For this review, take the finished solid that the model builds, in its own axes (mm). Face numbers are marked on the shaded views. Give positions to 0.01 mm unless a question says otherwise; leave off trailing zeros. Order: outer loops, then holes, each group sorted by start corner. A loop starts at its lowest first (then second) coordinate and runs counter-clockwise, first axis right, second up. Notation, with made-up numbers: (79.5, 35.25) - (126.5, 35.25) arc R30 ccw to (126.5, 66.25) - close; hole circle Ø5 at (-5, -29.75). An arc over 180 degrees is marked (long way). Put each result on its own line as item: value. Start each with the question number.
```python
from build123d import *

# Parameters (mm, degrees)
SKETCH1_R           = 12.35
BOSS_EXTRUDE1_DEPTH = 25
CIRPATTERN1_COUNT   = 4
SKETCH7_W           = 3.7
SKETCH7_H           = 1.9


with BuildPart() as part:
    # Sketch1 → Boss-Extrude1 (new body)
    with BuildSketch(Plane.XY):
        Circle(SKETCH1_R)
    extrude(amount=BOSS_EXTRUDE1_DEPTH)

    # Sketch2 → M4x0.7 Tapped Hole1 (revolve, cut)
    with BuildSketch(Plane(origin=(-0.784484958, 12.325059162, 10), x_dir=(-0.9979804989599389, -0.06352104923308127, 0), z_dir=(0, 0, 1))):
        Polygon((0, 0), (0, 9.991420021), (1.65, 9), (1.65, 0.85), (2.5, 0), align=None)
    m4x0_7_tapped_hole1 = revolve(axis=Axis((-1.187843621, 18.662235331, 10), (0.06352104923308129, -0.9979804989599389, 0)), mode=Mode.SUBTRACT)

    # CirPattern1: M4x0.7 Tapped Hole1 ×4 about axis
    cirpattern1_axis = Axis((0, 0, 25), (0, 0, -1))
    for i in range(1, CIRPATTERN1_COUNT):
        add(m4x0_7_tapped_hole1.rotate(cirpattern1_axis, i * 360 / CIRPATTERN1_COUNT), mode=Mode.SUBTRACT)

    # Sketch7 → Cut-Revolve1 (revolve, cut)
    with BuildSketch(Plane(origin=(0, 0, 0), x_dir=(0, 0, -1), z_dir=(1, 0, 0)), mode=Mode.PRIVATE) as cut_revolve1_sk:
        with Locations((-16.85, 11.4)):
            Rectangle(SKETCH7_W, SKETCH7_H)
    revolve(cut_revolve1_sk.sketch.rotate(Axis((0, 0, 25), (0, 0, -1)), 90), axis=Axis((0, 0, 25), (0, 0, -1)), mode=Mode.SUBTRACT)


solid = part.part
```
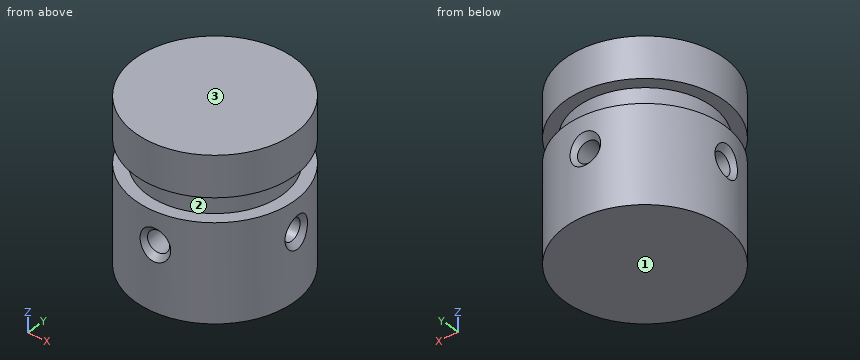
1. The part is to be moulded in two halves that separate along Z. For the marked faces 1, 2 and 3, say which applies: released by +Z, released by -Z, zero draft, split by the parting line, or undercut.
2. Clearance check with flat-ended pins moving along their axes: pin 1 (1.5 mm diameter, centred on x = -6.5, z = 7.5, fed in from -Y); pin 2 (1 mm diameter, centred on x = -9, z = 9.5, fed in from -Y); pin 3 (6 mm diameter, centred on x = 5.5, z = 17, fed in from +Y). State where each tip first meets the part, or that it passes through.
3. Wall thickness on line 1 (Z direction, x = 11, y = -5); line 2 (Z direction, x = -11, y = -0.5); line 3 (Z direction, x = 1, y = -4): over which ranges is each line inside the solid? List them lowest first. Write a range as from..to.
4. Add section A-A, the plane z = 18. Give the boundary of the cut face in (x, y).
Found:
1. face 1: released by -Z
1. face 2: undercut
1. face 3: released by +Z
2. pin 1: stops at y = -10.93
2. pin 2: stops at y = -8.96
2. pin 3: stops at y = 11.97
3. line 1: z = 0..15, 18.7..25
3. line 2: z = 0..8.36, 11.64..15, 18.7..25
3. line 3: z = 0..8.53, 11.47..25
4. outline: circle Ø20.9 at (0, 0)
